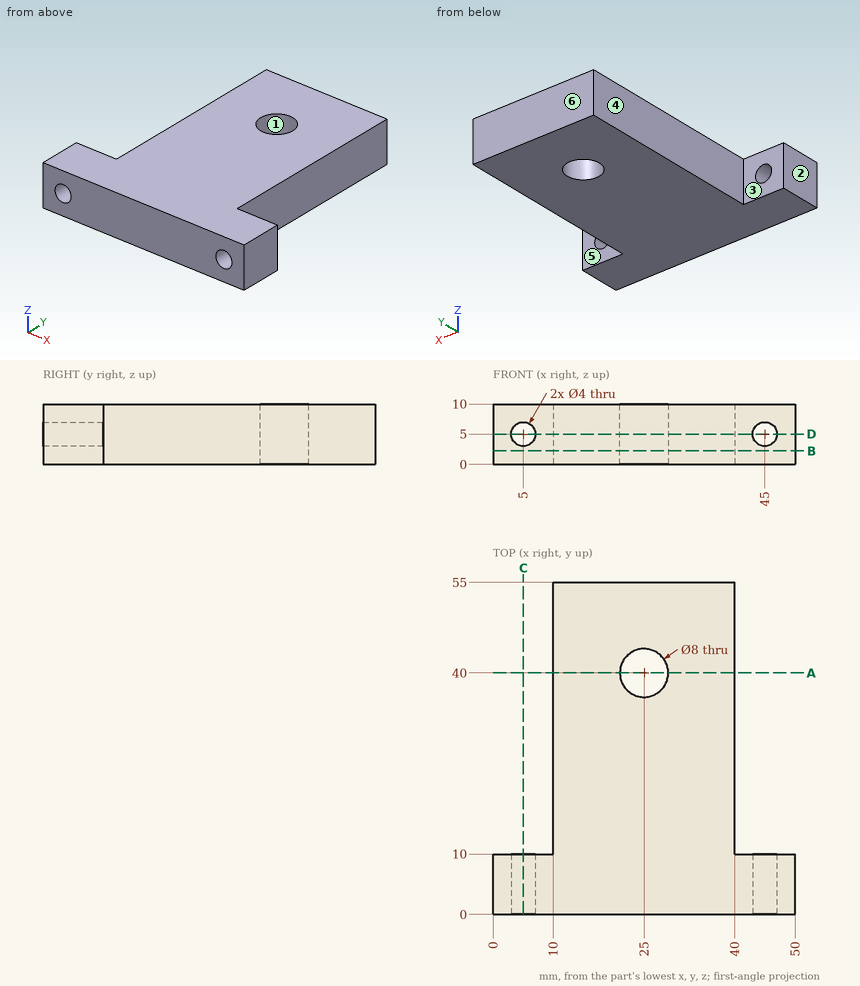
Design review of the part shown in the three views and the two pictorial views. Dimensions are in mm from the part's minimum x, y and z. A direction names the side the tool comes from. Give positions to 0.01 mm unless a question says otherwise; leave off trailing zeros. Order: outer loops, then holes, each group sorted by start corner. A loop starts at its lowest first (then second) coordinate and runs counter-clockwise, first axis right, second up. Notation, with made-up numbers: M 25,12 L 47,12 A27 cw 47,43 Z; hole C 57,72 d8. An arc over 180 degrees is marked long. Answer in a Markdown table with one row per item. Add a question column.
(1) For pin 1 (3 mm diameter, centred on x = 45.5, z = 3, fed in from +Y); pin 2 (1.5 mm diameter, centred on x = 35, z = 3.5, fed in from -Y); pin 3 (5 mm diameter, centred on y = 48, z = 3, fed in from -X), all flat-tipped, find the tip position at first contact; note any pin that passes through.
(2) Consider section B-B on z = 2.25. State the section outline as (x, y) points, and give its area (3 significant figures).
(3) Consider section D-D on z = 5. State the section outline as (x, y) points, and give its area (3 significant figures).
(4) For the marked faces 4, 5 and 6, list the 3-axis set-ups (+Z, -Z, +X, -X, +Y, -Y) from which the entire face can be reached by the end or side of a thin tool; tool diameter is ignored.
(5) Consider section A-A on y = 40. State the section outline as (x, z) points, and give its area (3 significant figures).
(6) Mouldability with a two-part tool opening along Y and no side actions: class the marked faces 1, 2 and 3 as +Y half, -Y half, draft (parallel to the pull), parting line (faces both ways), or undercut.
(7) Wall thickness on probe 1 along X at (y, z) = (2, 5); probe 2 along Y at (x, z) = (25, 2.75); probe 3 along X at (y, z) = (4, 3.75): over which ranges is each line inside the solid? List them lowest first. Write a range as [from, to].
(8) Consider section C-C on x = 5. State the section outline as (y, z) points, and give its area (3 significant figures).
Evaluation:
| question | item | result |
|---|---|---|
| 1 | pin 1 | stops at y = 10 |
| 1 | pin 2 | stops at y = 0 |
| 1 | pin 3 | stops at x = 10 |
| 2 | outline | M 0,0 L 50,0 L 50,10 L 40,10 L 40,55 L 10,55 L 10,10 L 0,10 Z; hole C 25,40 d8 |
| 2 | area | 1,800 mm^2 |
| 3 | outline | M 0,0 L 3,0 L 3,10 L 0,10 Z; M 7,0 L 43,0 L 43,10 L 40,10 L 40,55 L 10,55 L 10,10 L 7,10 Z; M 47,0 L 50,0 L 50,10 L 47,10 Z; hole C 25,40 d8 |
| 3 | area | 1,720 mm^2 |
| 4 | face 4 | +Z, -Z, -X, +Y |
| 4 | face 5 | +Z, -Z, +X, +Y |
| 4 | face 6 | +Z, -Z, +X, -X, +Y |
| 5 | outline | M 10,0 L 21,0 L 21,10 L 10,10 Z; M 29,0 L 40,0 L 40,10 L 29,10 Z |
| 5 | area | 220 mm^2 |
| 6 | face 1 | undercut |
| 6 | face 2 | draft |
| 6 | face 3 | +Y half |
| 7 | probe 1 | x = [0, 3], [7, 43], [47, 50] |
| 7 | probe 2 | y = [0, 36], [44, 55] |
| 7 | probe 3 | x = [0, 3.44], [6.56, 43.44], [46.56, 50] |
| 8 | outline | M 0,0 L 10,0 L 10,3 L 0,3 Z; M 0,7 L 10,7 L 10,10 L 0,10 Z |
| 8 | area | 60.0 mm^2 |
